Source: CAD feature listing. Evaluate the final solid. Frame: model axes, mm. A direction names the side the tool comes from. Give positions to 0.01 mm unless a question says otherwise; leave off trailing zeros. Write each loop counter-clockwise with the first axis right and the second up, starting at its lowest first coordinate (ties: lowest second). Pieces come first, ordered by that corner, then holes. Notation, with made-up numbers: (27, 30.5) -> (65, 30.5) arc R28 cw to (65, 52.5) -> close; hole circle Ø10 at (11.25, 69.5). An arc over 180 degrees is marked (long way). Write item = value, one per line.
from build123d import *

# Parameters (mm, degrees)
SKETCH3_R           = 2.5
BOSS_EXTRUDE2_DEPTH = 1
SKETCH4_R           = 2.5
SKETCH4_R_2         = 1.75
BOSS_EXTRUDE3_DEPTH = 2
SKETCH5_R           = 0.5
CUT_EXTRUDE1_DEPTH  = 2


with BuildPart() as part:
    # Sketch3 → Boss-Extrude2 (new body)
    with BuildSketch(Plane(origin=(0, 0, 0), x_dir=(1, 0, 0), z_dir=(0, 1, 0))):
        with BuildLine():
            Line((-1.5, 11), (-1.5, 2))
            ThreePointArc((-1.5, 2), (0, 2.5), (1.5, 2))
            Line((1.5, 2), (1.5, 11))
            ThreePointArc((1.5, 11), (0, 12.5), (-1.5, 11))
        make_face()
        Circle(SKETCH3_R)
    extrude(amount=BOSS_EXTRUDE2_DEPTH)

    # Sketch4 → Boss-Extrude3 (add)
    with BuildSketch(Plane(origin=(0, 1, 0), x_dir=(1, 0, 0), z_dir=(0, 1, 0))):
        with Locations(Location((0, 0, 0), (0, 0, 53.130102354))):
            Circle(SKETCH4_R)
        with Locations(Location((0, 0, 0), (0, 0, 270))):
            Circle(SKETCH4_R_2, mode=Mode.SUBTRACT)
    extrude(amount=BOSS_EXTRUDE3_DEPTH)

    # Sketch5 → Cut-Extrude1 (cut)
    with BuildSketch(Plane.XZ):
        with Locations(Location((0, -11, 0), (0, 0, 270))):
            Circle(SKETCH5_R)
    extrude(amount=-CUT_EXTRUDE1_DEPTH, mode=Mode.SUBTRACT)


solid = part.part
(1) Section query C-C (z = 1.25). Return loops of the section in (x, y).
Values follow:
outline = (-2.17, 0) -> (2.17, 0) -> (2.17, 3) -> (1.22, 3) -> (1.22, 1) -> (-1.22, 1) -> (-1.22, 3) -> (-2.17, 3) -> close
(2) Section query A-A (x = 0). Return loops of the section in (y, z).
Values follow:
outline = (0, -12.5) -> (1, -12.5) -> (1, -11.5) -> (0, -11.5) -> close; (0, -10.5) -> (1, -10.5) -> (1, -2.5) -> (3, -2.5) -> (3, -1.75) -> (1, -1.75) -> (1, 1.75) -> (3, 1.75) -> (3, 2.5) -> (0, 2.5) -> close
(3) First-contact query: pin 1 (0.5 mm diameter, centred on y = 0.5, z = -5, fed in from -X); pin 2 (3 mm diameter, centred on x = 0, z = 0, fed in from +Y). Flat tips, straight axial feed; report the tip coordinate or a pass-through.
Values follow:
pin_1 = -1.5
pin_2 = 1
(4) Section query D-D (x = 1.3). Return loops of the section in (y, z).
Values follow:
outline = (0, -11.75) -> (1, -11.75) -> (1, -2.14) -> (3, -2.14) -> (3, -1.17) -> (1, -1.17) -> (1, 1.17) -> (3, 1.17) -> (3, 2.14) -> (0, 2.14) -> close
(5) Access query for faces 1 (the face through (-1.71, 1.99, -0.38)), 2 (the face through (-1.5, 0.5, -6.6)), 3 (the face through (1.5, 0.5, -6.4)), 4 (the face through (0, 0, -5)). Directions: +Z, -Z, +X, -X, +Y, -Y. A direction counts if a zero-diameter tool reaches every point of the face in a straight line with its end or side. Return the directions, or none.
Values follow:
face_1 = +Y
face_2 = -Z, -X, +Y, -Y
face_3 = -Z, +X, +Y, -Y
face_4 = +Z, -Z, +X, -X, -Y
(6) Material intervals for line 1 (X direction, y = 0.5, z = -11); line 2 (X direction, y = 0.9, z = -6.5); line 3 (Y direction, x = -0.35, z = -8.5), sorted ascending.
Values follow:
line_1 = -1.5 to -0.5, 0.5 to 1.5
line_2 = -1.5 to 1.5
line_3 = 0 to 1
(7) Section query B-B (y = 0.5). Return loops of the section in (x, z), plus the area to 3 significant figures.
Values follow:
outline = (-1.5, -11) arc R1.5 ccw to (1.5, -11) -> (1.5, -2) arc R2.5 ccw (long way) to (-1.5, -2) -> close; hole circle Ø1 at (0, -11)
area = 48.4 mm2
(8) Pull-direction query (Z, two-part tool) for faces 5 (the face through (0, 0.5, -12.5)), 6 (the face through (0, 1, 0)), 7 (the face through (0, 1, -7)); classes: pulls with the +Z half, pulls with the -Z half, needs draft (parallel to the pull), parting line crosses it, or undercut.
Values follow:
face_5 = pulls with the -Z half
face_6 = undercut
face_7 = needs draft
